The model under review builds one solid part; all positions refer to its coordinate system, in mm. A direction names the side the tool comes from. Coordinates: 2 decimals unless noted, no trailing zeros. Write each loop counter-clockwise with the first axis right and the second up, starting at its lowest first coordinate (ties: lowest second). Pieces come first, ordered by that corner, then holes. Notation, with made-up numbers: (41.25, -13) - (79.25, -13) arc R13 cw to (79.25, 10) - close; hole circle Ø10 at (3.25, 85). An arc over 180 degrees is marked (long way). Return JSON: item names as keys, results as strings. Group by question number.
(1) For pin 1 Ø4 at (x, y) = (2.5, -119) entering from +Z; pin 2 Ø2 at (x, y) = (-4, -211) entering from -Z; pin 3 Ø6 at (x, z) = (5.5, 4.5) entering from -Y, all flat-tipped, find the tip position at first contact; note any pin that passes through.
(2) Tool access review of faces 1 (the face through (-0.59, -121.57, 4.46)), 2 (the face through (0, 10, 0)): name each direction out of +Z, -Z, +X, -X, +Y, -Y from which nothing blocks a thin tool from reaching the whole face with its end or side.
(3) We need section B-B on z = 0. State the section outline as (x, y) points, then the cut area to 3 significant figures.
(4) We need section A-A on x = 0. State the section outline as (y, z) points.
(5) To check wall thickness, follow L1, parallel to Y at x = -4.75, z = 3.75; L2, parallel to X at y = -15.5, z = -0.5; L3, parallel to Z at x = 0, y = -141. State the ranges of each line that lie inside material, in increasing order. Write a range as from..to.
(6) We need section C-C on y = -10. State the section outline as (x, z) points, then the cut area to 3 significant figures.
```python
from build123d import *

# Parameters (mm, degrees)
F0_R     = 4.5
F1_DEPTH = 248
F2_R     = 7.5
F3_DEPTH = 10
F4_SIZE  = 1.4


with BuildPart() as f1:
    # F0 (on Front) → F1 (new body)
    with BuildSketch(Plane.XZ):
        Circle(F0_R)
    extrude(amount=F1_DEPTH)

    # F2 (on face) → F3 (join)
    with BuildSketch(Plane(origin=(0, 0, 0), x_dir=(-1, 0, 0), z_dir=(0, 1, 0))):
        Circle(F2_R)
    extrude(amount=F3_DEPTH)

    # F4
    f4_edges = [f1.edges().sort_by_distance(p)[0] for p in [
        (-4.5, -248, 0),
    ]]
    chamfer(f4_edges, length=F4_SIZE)


solid = f1.part
```
Ans:
{
 "1": {"pin 1": "z = 4.47", "pin 2": "z = -3.35", "pin 3": "y = -246.99"},
 "2": {"face 1": "-Y", "face 2": "+Z, -Z, +X, -X, +Y"},
 "3": {"outline": "(-7.5, 0) - (-4.5, 0) - (-4.5, -246.6) - (-3.1, -248) - (3.1, -248) - (4.5, -246.6) - (4.5, 0) - (7.5, 0) - (7.5, 10) - (-7.5, 10) - close", "area": "2,380 mm²"},
 "4": {"outline": "(-248, -3.1) - (-246.6, -4.5) - (0, -4.5) - (0, -7.5) - (10, -7.5) - (10, 7.5) - (0, 7.5) - (0, 4.5) - (-246.6, 4.5) - (-248, 3.1) - close"},
 "5": {"L1": "0..10", "L2": "-4.47..4.47", "L3": "-4.5..4.5"},
 "6": {"outline": "circle Ø9 at (0, 0)", "area": "63.6 mm²"}
}
